Read the model definition and answer for the solid it produces. Units are mm, in the model's axes. Face numbers are marked on the shaded views. A direction names the side the tool comes from. Coordinates: 2 decimals unless noted, no trailing zeros. Write each loop counter-clockwise with the first axis right and the second up, starting at its lowest first coordinate (ties: lowest second). Pieces come first, ordered by that corner, then holes. Notation, with made-up numbers: (53.25, 39.25) -> (111.25, 39.25) arc R18 ccw to (111.25, 66.25) -> close; hole circle Ø4 at (-4.75, 25.5). An arc over 180 degrees is marked (long way). Write item = value, one per line. Start each with the question number.
1) Find the intervals of material crossed by line 1 along Z through (x, y) = (24.5, -8.75); line 2 along Z through (x, y) = (6, -9.5); line 3 along Z through (x, y) = (2.5, -5), in increasing order. Write a range as from..to.
2) Section A-A (x = 33) is taken. Determine the outline of the cut face in (y, z), plus the area to 3 significant figures.
3) Section D-D (z = -20.5) is taken. Determine the outline of the cut face in (x, y).
4) A tool of negligible diameter and unlimited length cuts with its end or side. For the marked faces 1, 2 and 3, from which of +Z, -Z, +X, -X, +Y, -Y can it reach the whole face along a straight path? Write none if from no direction.
5) For a pull along Z with two mould halves and no side action, classify the marked faces 4, 5 and 6 as released by +Z, released by -Z, zero draft, split by the parting line, or undercut.
6) Section B-B (x = 4.5) is taken. Determine the outline of the cut face in (y, z), plus the area to 3 significant figures.
7) Flat-ended cylindrical pins translate along their axes: pin 1 Ø3.5 at (x, y) = (2, -6) entering from +Z; pin 2 Ø0.6 at (y, z) = (-6, 1) entering from -X; pin 3 Ø3 at (y, z) = (-5.5, -6) entering from -X. Find the tip coordinate at first contact, or state that the pin passes through.
8) Section C-C (y = -9.5) is taken. Determine the outline of the cut face in (x, z), plus the area to 3 significant figures.
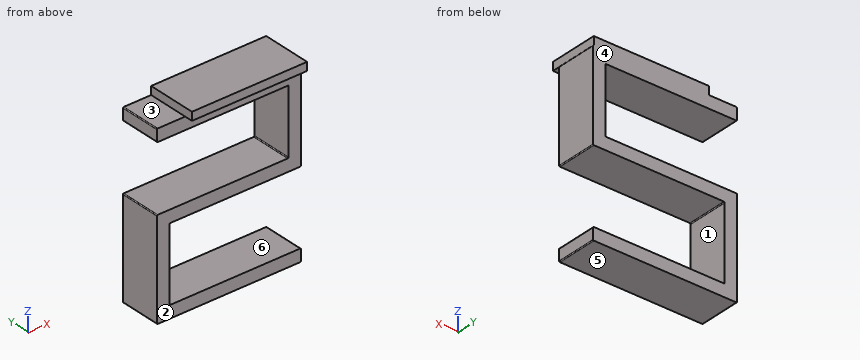
from build123d import *

# Parameters (mm, degrees)
F1_DEPTH = 10
F2_R     = 0.2
F3_R     = 0.2
F4_W     = 28
F4_H     = 2
F5_DEPTH = 25
F6_DEPTH = 13
F7_DEPTH = 12
F8_DEPTH = 1


with BuildPart() as f1:
    # F0 (on Front) → F1 (new body)
    with BuildSketch(Plane.XZ):
        Polygon((35, 0), (0, 0), (0, -3), (32, -3), (32, -18.9999993891), (0, -18.9999993891), (0, -43), (35, -43), (35, -39.9999991059), (3, -39.9999991059), (3, -21.9999998808), (35, -21.9999998808), align=None)
    extrude(amount=F1_DEPTH)

    # F2
    f2_edges = [f1.edges().sort_by_distance(p)[0] for p in [
        (35, -5, 0),
        (32, -5, -3),
        (35, -5, -22),
        (32, -5, -18.999999),
    ]]
    fillet(f2_edges, radius=F2_R)

    # F3
    f3_edges = [f1.edges().sort_by_distance(p)[0] for p in [
        (3, -5, -39.999999),
        (35, -5, -39.999999),
        (35, -5, -43),
        (0, -5, -43),
        (3, -5, -22),
        (0, -5, -18.999999),
        (0, -5, 0),
        (0, -5, -3),
    ]]
    fillet(f3_edges, radius=F3_R)

    # F4 (on Front) → F5 (join)
    with BuildSketch(Plane.XZ):
        with Locations((20.8566440605, 1)):
            Rectangle(F4_W, F4_H)
    extrude(amount=F5_DEPTH)

    # F6 (add): a face of the model
    f6_faces = [f1.faces().sort_by_distance(p)[0] for p in [
        (20.8566440605, -25, 1),
    ]]
    extrude(f6_faces, amount=-F6_DEPTH)

    # F7 (cut): a face of the model
    f7_faces = [f1.faces().sort_by_distance(p)[0] for p in [
        (20.8566440605, -25, 1),
    ]]
    extrude(f7_faces, amount=-F7_DEPTH, mode=Mode.SUBTRACT)

    # F8 (cut): a face of the model
    f8_faces = [f1.faces().sort_by_distance(p)[0] for p in [
        (20.8566440605, -13, 1),
    ]]
    extrude(f8_faces, amount=-F8_DEPTH, mode=Mode.SUBTRACT)


solid = f1.part
Answer key:
q1.line_1 = -43..-40, -22..-19, -3..2
q1.line_2 = -43..-40, -22..-19, -3..0
q1.line_3 = -43..-19, -3..0
q2.outline = (-12, 0) -> (-10, 0) -> (-10, -22) -> (0, -22) -> (0, 2) -> (-12, 2) -> close; (-10, -43) -> (0, -43) -> (0, -40) -> (-10, -40) -> close
q2.area = 274 mm^2
q3.outline = (0, -10) -> (35, -10) -> (35, 0) -> (0, 0) -> close
q4.face_1 = +X, +Y, -Y
q4.face_2 = -Z, +X, -X, -Y
q4.face_3 = +Z, -X, +Y, -Y
q5.face_4 = zero draft
q5.face_5 = released by -Z
q5.face_6 = undercut
q6.outline = (-10, -43) -> (0, -43) -> (0, -40) -> (-10, -40) -> close; (-10, -22) -> (0, -22) -> (0, -19) -> (-10, -19) -> close; (-10, -3) -> (0, -3) -> (0, 0) -> (-10, 0) -> close
q6.area = 90.0 mm^2
q7.pin_1 = 0
q7.pin_2 = 6.86
q7.pin_3 = 32
q8.outline = (0, -42.8) arc R0.2 ccw to (0.2, -43) -> (34.8, -43) arc R0.2 ccw to (35, -42.8) -> (35, -40.2) arc R0.2 ccw to (34.8, -40) -> (3.2, -40) arc R0.2 cw to (3, -39.8) -> (3, -22.2) arc R0.2 cw to (3.2, -22) -> (34.8, -22) arc R0.2 ccw to (35, -21.8) -> (35, -0.2) arc R0.2 ccw to (34.8, 0) -> (34.86, 0) -> (34.86, 2) -> (6.86, 2) -> (6.86, 0) -> (0.2, 0) arc R0.2 ccw to (0, -0.2) -> (0, -2.8) arc R0.2 ccw to (0.2, -3) -> (31.8, -3) arc R0.2 cw to (32, -3.2) -> (32, -18.8) arc R0.2 cw to (31.8, -19) -> (0.2, -19) arc R0.2 ccw to (0, -19.2) -> close
q8.area = 473 mm^2
